Read the model definition and answer for the solid it produces. Units are mm, in the model's axes. Round coordinates to 2 decimals unless told otherwise and drop trailing zeros. Write each loop counter-clockwise with the first axis right and the second up, starting at its lowest first coordinate (ties: lowest second). Pieces come first, ordered by that corner, then holes. Notation, with made-up numbers: (-18.5, 28.5) - (40.5, 28.5) arc R16 cw to (40.5, 35.5) - close; hole circle Ø3 at (19.5, 55.25). An arc over 180 degrees is marked (long way). Answer as CSV lines item,"result". Start each with the question number.
1) Find section B-B on y = 1.5. State how many separate pieces and enclosed holes the cut face has, then the cut area to 3 significant figures.
2) Find section A-A on z = -0.95. Determine the outline of the cut face in (x, y).
3) Consider line 1 along Y through (x, z) = (0, 0.2); line 2 along X through (y, z) = (1.5, -0.05); line 3 along Y through (x, z) = (-9, 0.6). Determine where each line is inside the solid, lowest interval first.
4) Each of these flat-tipped pins is pushed along its axis until it touches: pin 1 (0.5 mm diameter, centred on x = -0.5, z = 0, fed in from -Y); pin 2 (10 mm diameter, centred on x = -4.5, y = 2.5, fed in from +Z); pin 3 (3 mm diameter, centred on x = 0, y = 2.5, fed in from -Z). Where does it stop, or does it pass through?
from build123d import *

# Parameters (mm, degrees)
SWEEP1_PROFILE_R        = 1.5
SKETCH7_R               = 0.5
CUT_EXTRUDE1_DEPTH      = 2.5000001
CUT_EXTRUDE1_DEPTH_BACK = 2.5000001
CUT_EXTRUDE10_DEPTH     = 2


with BuildPart() as part:
    # Sweep1: sweep along a path in Sketch2
    with BuildLine(Plane.XY) as sweep1_path:
        Line((0, 0), (0, 5))
        ThreePointArc((0, 5), (-5.724351322, 11.882784353), (-13.535062985, 7.508575647))
        Line((-13.535062985, 7.508575647), (-23.465153554, -18.360194706))
        ThreePointArc((-23.465153554, -18.360194706), (-22.520539139, -25.081475515), (-16.32000037, -27.842133239))
        Line((-16.32000037, -27.842133239), (-6.389909801, -26.973362887))
        ThreePointArc((-6.389909801, -26.973362887), (-1.839058642, -24.729131453), (0, -20))
        Line((0, -20), (0, -15))
    # Sweep1 profile (on start of the path) → Sweep1 (sweep)
    with BuildSketch(Plane.ZX):
        Circle(SWEEP1_PROFILE_R)
    sweep(path=sweep1_path.line)

    # Sketch7 → Cut-Extrude1 (cut, two sides)
    with BuildSketch(Plane.XY) as cut_extrude1_sk:
        with Locations((0, 1.5)):
            Circle(SKETCH7_R)
        Polygon((1.5, -15), (-3.26701437, -19), (-3.26701437, -15), align=None)
    extrude(amount=CUT_EXTRUDE1_DEPTH, mode=Mode.SUBTRACT)
    extrude(cut_extrude1_sk.sketch, amount=-CUT_EXTRUDE1_DEPTH_BACK, mode=Mode.SUBTRACT)

    # Sketch9 → Cut-Extrude10 (cut, symmetric)
    with BuildSketch(Plane(origin=(0, 0, 0), x_dir=(0, 0, -1), z_dir=(1, 0, 0))):
        with BuildLine():
            Line((0.5, 0), (0.5, 3.267949192))
            ThreePointArc((0.5, 3.267949192), (0.767949192, 4.267949192), (1.5, 5))
            Line((1.5, 5), (1.5, 0))
            Line((1.5, 0), (0.5, 0))
        make_face()
        with BuildLine():
            Line((0.500000276, -15), (0.500000276, -18.267949352))
            ThreePointArc((0.500000276, -18.267949352), (0.767949389, -19.267949214), (1.5, -20))
            Line((1.5, -20), (1.5, -15))
            Line((1.5, -15), (0.500000276, -15))
        make_face()
    cut_extrude10 = extrude(amount=CUT_EXTRUDE10_DEPTH, both=True, mode=Mode.SUBTRACT)

    # Mirror1: Cut-Extrude10 across plane
    add(cut_extrude10.mirror(Plane.XY), mode=Mode.SUBTRACT)


solid = part.part
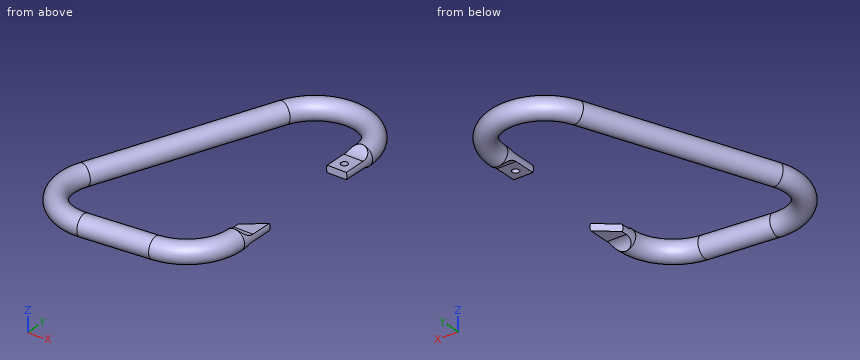
Check values:
1,separate pieces,"3"
1,enclosed holes,"0"
1,area,"9.51 mm^2"
2,outline,"(-24.55, -17.94) arc R8.16 ccw to (-16.22, -29) - (-6.29, -28.13) arc R8.16 ccw to (1.16, -20) - (1.16, -19.53) - (-1.16, -19.53) - (-1.16, -20) arc R5.84 cw to (-6.49, -25.82) - (-16.42, -26.69) arc R5.84 cw to (-22.38, -18.78) - (-12.45, 7.09) arc R5.84 cw to (-1.16, 5) - (-1.16, 4.53) - (1.16, 4.53) - (1.16, 5) arc R8.16 ccw to (-14.62, 7.92) - close"
3,line 1,"y = -24.8 to -16.26, 0 to 1, 2 to 9.8"
3,line 2,"x = -17.45 to -14.24, -1.5 to -0.5, 0.5 to 1.5"
3,line 3,"y = -28.58 to -25.82, 10.26 to 13.13"
4,pin 1,"stops at y = -25.76"
4,pin 2,"stops at z = 1.49"
4,pin 3,"stops at z = -0.64"
